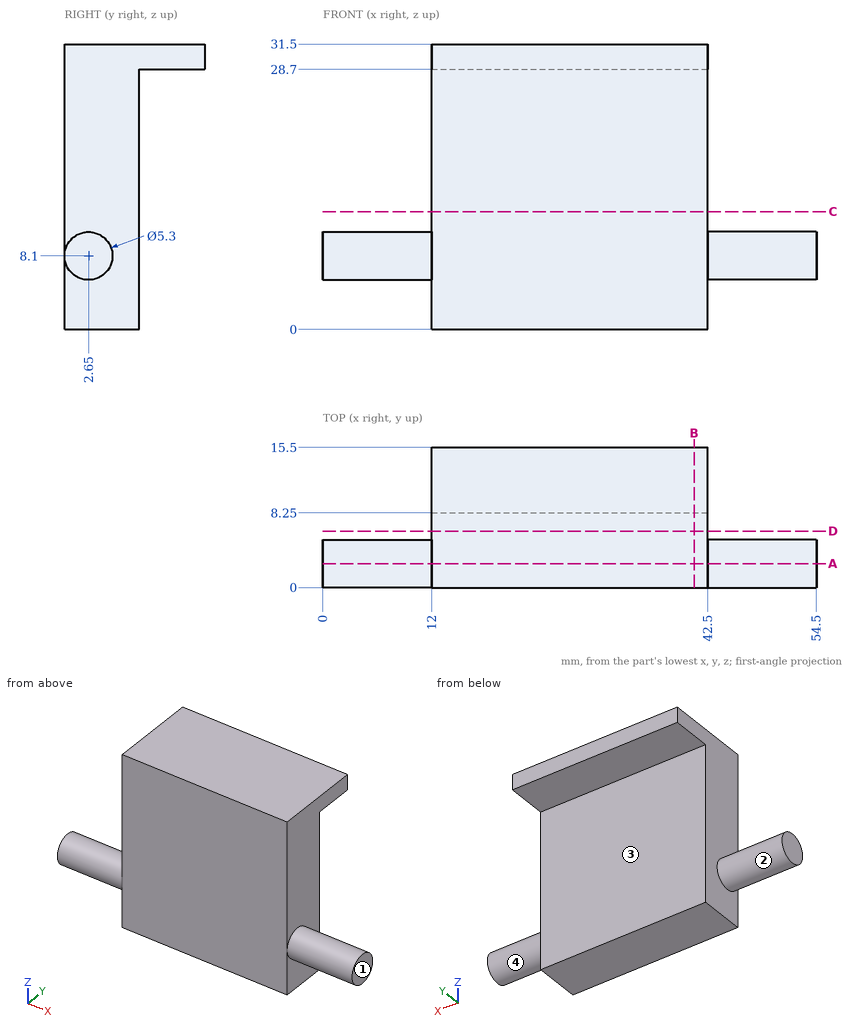
Part print with two shaded views. Sizes in mm from the minimum x, y, z corner. A direction names the side the tool comes from. Round coordinates to 2 decimals unless told otherwise and drop trailing zeros. Write each loop counter-clockwise with the first axis right and the second up, starting at its lowest first coordinate (ties: lowest second). Pieces come first, ordered by that corner, then holes. Notation, with made-up numbers: (6, 39) - (65, 39) arc R23 cw to (65, 66) - close; hole circle Ø1 at (-7.75, 38.25). An arc over 180 degrees is marked (long way). Answer as CSV lines item,"result".
Q1. Cut at C-C (z = 13). Write the cut outline in (x, y), and give its area (3 significant figures).
Report:
outline,"(12, 0) - (42.5, 0) - (42.5, 8.25) - (12, 8.25) - close"
area,"252 mm^2"
Q2. Cut at B-B (x = 41). Write the cut outline in (y, z).
Report:
outline,"(0, 0) - (8.25, 0) - (8.25, 28.7) - (15.5, 28.7) - (15.5, 31.5) - (0, 31.5) - close"
Q3. Drop flat-ended pins along their axis: pin 1 (4 mm diameter, centred on x = 20, z = 21, fed in from +Y); pin 2 (2 mm diameter, centred on y = 3, z = 15, fed in from +X); pin 3 (3.5 mm diameter, centred on x = 29.5, y = 12.5, fed in from -Z). Give the stop position or say it passes through.
Report:
pin 1,"stops at y = 8.25"
pin 2,"stops at x = 42.5"
pin 3,"stops at z = 28.7"
Q4. Cut at D-D (y = 6.25). Write the cut outline in (x, z).
Report:
outline,"(12, 0) - (42.5, 0) - (42.5, 31.5) - (12, 31.5) - close"
Q5. Cut at A-A (y = 2.65). Write the cut outline in (x, z), and give its area (3 significant figures).
Report:
outline,"(0, 5.45) - (12, 5.45) - (12, 0) - (42.5, 0) - (42.5, 5.45) - (54.5, 5.45) - (54.5, 10.75) - (42.5, 10.75) - (42.5, 31.5) - (12, 31.5) - (12, 10.75) - (0, 10.75) - close"
area,"1,090 mm^2"
Q6. Drill centre lines: probe 1 along Z at (x, y) = (29, 11.5); probe 2 along X at (y, z) = (7, 11); probe 3 along Y at (x, z) = (35, 16.5). Where is each one in solid material? Low to high. Write a range as [from, to].
Report:
probe 1,"z = [28.7, 31.5]"
probe 2,"x = [12, 42.5]"
probe 3,"y = [0, 8.25]"
Q7. Tool access for the marked faces 1, 2, 3 and 4: list every direction of +Z, -Z, +X, -X, +Y, -Y with a clear straight run to the whole face (end or side of a thin tool).
Report:
face 1,"+Z, -Z, +X, +Y, -Y"
face 2,"-X"
face 3,"-Z, +X, -X, +Y"
face 4,"+X"
